For this review, take the finished solid that the model builds, in its own axes (mm). A direction names the side the tool comes from. Give positions to 0.01 mm unless a question says otherwise; leave off trailing zeros. Loops run counter-clockwise (first coordinate to the right, second up) from the corner with the lowest first, then second, coordinate; pieces in that order, holes last. Notation, with made-up numbers: (27, 56) -> (65, 56) arc R18 ccw to (65, 83) -> close; hole circle Ø4 at (53, 28). An arc over 180 degrees is marked (long way). One line per question, with ' | ' between items. Start each with the question number.
(1) Tool access review of faces 1 (the cylindrical face through (-23.84, -42.88, 28.54)), 2 (the flat face through (-23, -49, 63.5)): name each direction out of +Z, -Z, +X, -X, +Y, -Y from which nothing blocks a thin tool from reaching the whole face with its end or side.
(2) Draft analysis for pull direction Y (two halves, no side actions). For faces 3 (the cylindrical face through (-25.355, -47.029, 32.194)), 4 (the flat face through (-22, -46, 0)), 5 (the conical face through (-22.34, -50.48, 65.56)), state which applies: +Y half, -Y half, draft (parallel to the pull), parting line (faces both ways), or undercut.
(3) Wall thickness on probe 1 along X at (y, z) = (-49, 50); probe 2 along Y at (x, z) = (-23, 5); probe 3 along Y at (x, z) = (-24.25, 53): over which ranges is each line inside the solid? List them lowest first.
(4) Insertion check: P1, Ø1.9, axis at x = -23, y = -48.5, coming from the -Z side; P2, Ø2, axis at y = -44.5, z = 9, coming from the +X side; P3, Ø1, axis at x = -19.5, z = 40, coming from the +Y side. Each pin has a flat end and moves straight along its axis. Give the tip position at first contact, or say it passes through.
(5) Consider section A-A (z = 6.5). Write out the cut boundary in (x, y) (3 decimals), and give its area (3 significant figures).
from build123d import *

# Parameters (mm, degrees)
F0_R     = 6.35
F1_DEPTH = 63.5
F3_R     = 6.35
F4_DEPTH = 3.81
F5_D     = 6.35
F5_DEPTH = 63.5
F5_TIP   = 1.9077324654
F6_SIZE2 = 7.567635313
F6_SIZE  = 6.35
F7_R     = 5.08


with BuildPart() as f1:
    # F0 (on Top) → F1 (new body)
    with BuildSketch(Plane.XY):
        with Locations((-23.0151098222, -49.1751506925)):
            Circle(F0_R)
    extrude(amount=F1_DEPTH)

    # F3 (on face) → F4 (join)
    with BuildSketch(Plane.XY.offset(63.5)):
        with Locations((-23.0151098222, -49.1751506925)):
            Circle(F3_R)
    extrude(amount=F4_DEPTH)

    # F5 (one way)
    with BuildSketch(Plane.XY.offset(63.5)):
        with Locations((-23.0151098222, -49.1751506925)):
            Circle(F5_D / 2)
    extrude(amount=-F5_DEPTH, mode=Mode.SUBTRACT)
    with Locations(Plane.XY.offset(63.5)):
        with Locations((-23.0151098222, -49.1751506925)):
            with Locations((0, 0, -(F5_DEPTH + F5_TIP / 2))):  # 118° drill point
                Cone(0, F5_D / 2, F5_TIP, mode=Mode.SUBTRACT)

    # F6
    f6_edges = [f1.edges().sort_by_distance(p)[0] for p in [
        (-29.36511, -49.175151, 67.31),
    ]]
    f6_side = f1.faces().sort_by_distance((-23.01511, -49.175151, 67.31))[0]
    chamfer(f6_edges, length=F6_SIZE, length2=F6_SIZE2, reference=f6_side)

    # F7
    f7_edges = [f1.edges().sort_by_distance(p)[0] for p in [
        (-29.36511, -49.175151, 59.742365),
    ]]
    fillet(f7_edges, radius=F7_R)


solid = f1.part
A:
1) face 1: +Z, -Z | face 2: -Z
2) face 3: undercut | face 4: draft | face 5: parting line
3) probe 1: x = -29.36 to -26.19, -19.84 to -16.67 | probe 2: y = -55.53 to -52.35, -46 to -42.83 | probe 3: y = -55.4 to -52.1, -46.25 to -42.95
4) P1: stops at z = 63.5 | P2: stops at x = -17.84 | P3: stops at y = -43.59
5) outline: circle Ø12.7 at (-23.015, -49.175); hole circle Ø6.35 at (-23.015, -49.175) | area: 95.0 mm^2
